```python
from build123d import *

# Parameters (mm, degrees)
F0_R     = 75
F0_R_2   = 7.5
F0_R_3   = 20
F1_DEPTH = 2
F2_R     = 20
F2_R_2   = 7.5
F3_DEPTH = 15


with BuildPart() as f1:
    # F0 (on Front) → F1 (new body)
    with BuildSketch(Plane.XZ):
        Circle(F0_R)
        with Locations((-47.6313972081, -27.5)):
            Circle(F0_R_2, mode=Mode.SUBTRACT)
        with Locations((0, -55)):
            Circle(F0_R_2, mode=Mode.SUBTRACT)
        with Locations((47.6313972081, -27.5)):
            Circle(F0_R_2, mode=Mode.SUBTRACT)
        with Locations((-47.6313972081, 27.5)):
            Circle(F0_R_2, mode=Mode.SUBTRACT)
        Circle(F0_R_3, mode=Mode.SUBTRACT)
        with Locations((47.6313972081, 27.5)):
            Circle(F0_R_2, mode=Mode.SUBTRACT)
        with Locations((0, 55)):
            Circle(F0_R_2, mode=Mode.SUBTRACT)
    extrude(amount=F1_DEPTH)

    # F2 (on face) → F3 (join)
    with BuildSketch(Plane(origin=(0, 0, 0), x_dir=(-1, 0, 0), z_dir=(0, 1, 0))):
        Circle(F2_R)
        Circle(F2_R_2, mode=Mode.SUBTRACT)
    extrude(amount=-F3_DEPTH)


solid = f1.part
```
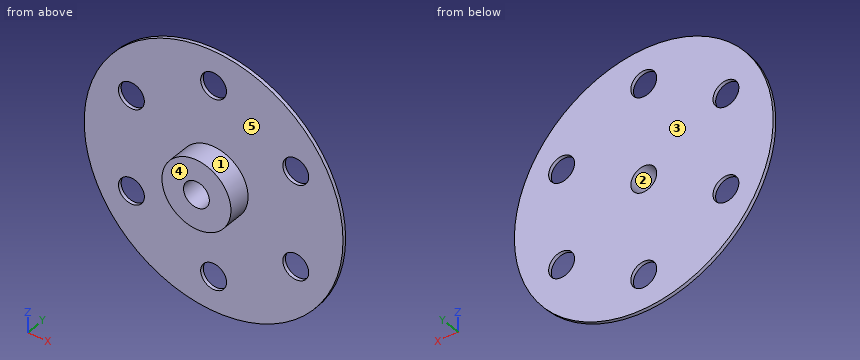
Can you work these out from the model? Positions are in its coordinate system, mm. Face numbers are marked on the shaded views. A direction names the side the tool comes from. Coordinates: 2 decimals unless noted, no trailing zeros. Order: outer loops, then holes, each group sorted by start corner. A loop starts at its lowest first (then second) coordinate and runs counter-clockwise, first axis right, second up.
1. If we section it at B-B (x = 0): Please give me the cut outline in (y, z), then the cut area to 3 significant figures.
2. If we section it at C-C (x = 47): Please give me the cut outline in (y, z).
3. I'm going to push flat-ended pins straight in: pin 1 (1.5 mm diameter, centred on x = -0.5, y = -2.5, fed in from -Z); pin 2 (24 mm diameter, centred on x = 0, z = 55, fed in from -Y); pin 3 (13.5 mm diameter, centred on x = 47.63, z = 27.5, fed in from +Y); pin 4 (3 mm diameter, centred on y = -10, z = -5.5, fed in from -X). Where does each tip first touch, or does it pass through?
4. If we section it at A-A (z = 0): Please give me the cut outline in (x, y).
5. If we section it at D-D (y = -8.5): Please give me the cut outline in (x, z), then the cut area to 3 significant figures.
6. Thinking about a two-plate mould opening in Z: for the marked faces 1, 2 and 3, which applies, +Z half, -Z half, draft (parallel to the pull), parting line (faces both ways), or undercut?
7. For the marked faces 4 and 5, which set-ups out of +Z, -Z, +X, -X, +Y, -Y let a thin tool reach every point of the face, with its end or its side?
8. I need wall thicknesses on line 1 (Z direction, x = 0, y = -1.1); line 2 (Y direction, x = 24.5, z = -44.5); line 3 (Z direction, x = 0, y = -6.5). Which ranges of each line are inside material? Lowest first, please.
Entries:
1. outline: (-15, -20) - (-2, -20) - (-2, -47.5) - (0, -47.5) - (0, -7.5) - (-15, -7.5) - close; (-15, 7.5) - (0, 7.5) - (0, 47.5) - (-2, 47.5) - (-2, 20) - (-15, 20) - close; (-2, -75) - (0, -75) - (0, -62.5) - (-2, -62.5) - close; (-2, 62.5) - (0, 62.5) - (0, 75) - (-2, 75) - close
1. area: 535 mm2
2. outline: (-2, -58.45) - (0, -58.45) - (0, -34.97) - (-2, -34.97) - close; (-2, -20.03) - (0, -20.03) - (0, 20.03) - (-2, 20.03) - close; (-2, 34.97) - (0, 34.97) - (0, 58.45) - (-2, 58.45) - close
3. pin 1: stops at z = -75
3. pin 2: stops at y = -2
3. pin 3: passes through
3. pin 4: stops at x = -19.6
4. outline: (-75, -2) - (-20, -2) - (-20, -15) - (-7.5, -15) - (-7.5, 0) - (-75, 0) - close; (7.5, -15) - (20, -15) - (20, -2) - (75, -2) - (75, 0) - (7.5, 0) - close
5. outline: circle Ø40 at (0, 0); hole circle Ø15 at (0, 0)
5. area: 1,080 mm2
6. face 1: parting line
6. face 2: undercut
6. face 3: draft
7. face 4: +Z, -Z, +X, -X, -Y
7. face 5: -Y
8. line 1: z = -75 to -62.5, -47.5 to -7.5, 7.5 to 47.5, 62.5 to 75
8. line 2: y = -2 to 0
8. line 3: z = -20 to -7.5, 7.5 to 20
